Here's the drawing with two shaded views (mm, measured from the low corner). I have some questions. A direction names the side the tool comes from. Round coordinates to 2 decimals unless told otherwise and drop trailing zeros. Loops run counter-clockwise (first coordinate to the right, second up) from the corner with the lowest first, then second, coordinate; pieces in that order, holes last. Notation, with made-up numbers: (70, 2) -> (84, 2) arc R20 ccw to (84, 20) -> close; hole circle Ø2 at (84.5, 67.5). An arc over 180 degrees is marked (long way). Use a Markdown table: item, result.
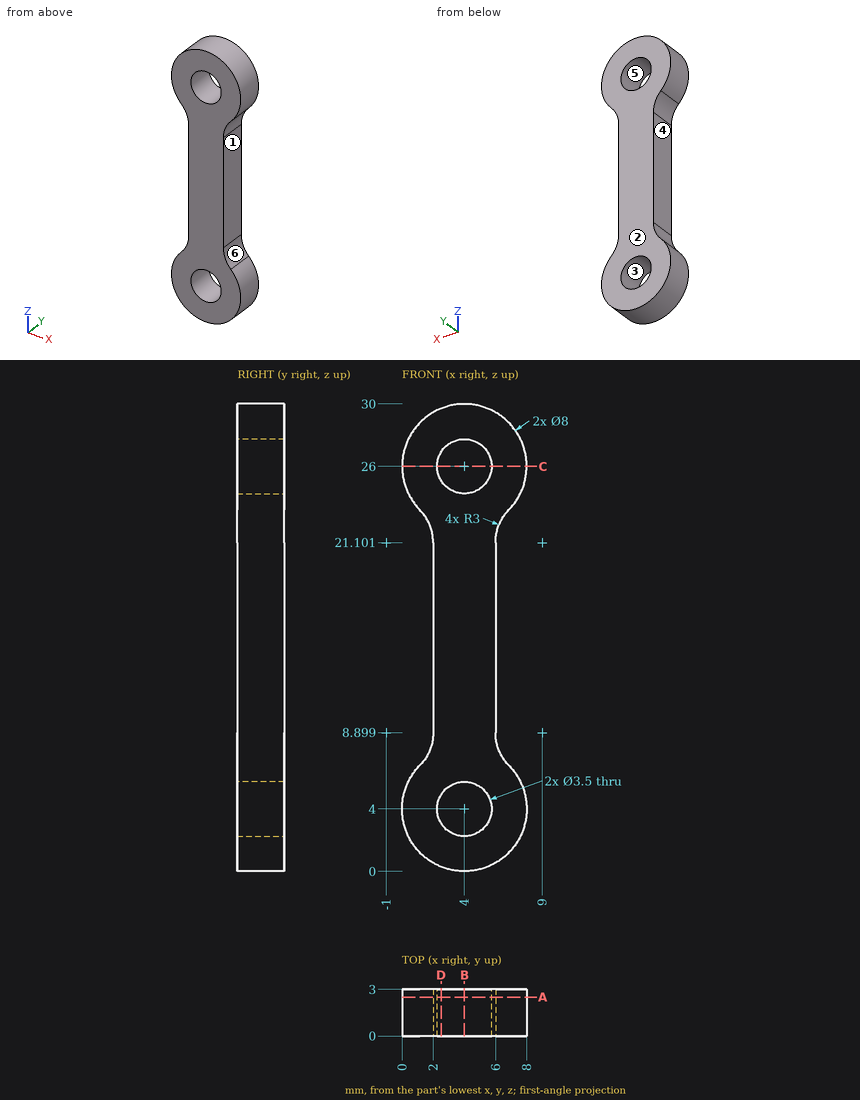
1. If we mould it in two halves opening along Z, with no side actions, what happens to the marked faces 1, 2 and 3? For each: +Z half, -Z half, draft (parallel to the pull), parting line (faces both ways), or undercut.
Answer sheet:
| item | result |
|---|---|
| face 1 | undercut |
| face 2 | draft |
| face 3 | undercut |
2. Which directions (+Z, -Z, +X, -X, +Y, -Y) give clear straight access to the entire face, cutting with the end or side of a thin tool? Please do the marked faces 4, 5 and 6.
Answer sheet:
| item | result |
|---|---|
| face 4 | -X, +Y, -Y |
| face 5 | +Y, -Y |
| face 6 | +X, +Y, -Y |
3. I want a section at C-C (z = 26). Please give me the cut outline in (x, y).
Answer sheet:
| item | result |
|---|---|
| outline | (0, 0) -> (2.25, 0) -> (2.25, 3) -> (0, 3) -> close; (5.75, 0) -> (8, 0) -> (8, 3) -> (5.75, 3) -> close |
4. I want a section at A-A (y = 2.5). Please give me the cut outline in (x, z).
Answer sheet:
| item | result |
|---|---|
| outline | (1.14, 6.8) arc R4 ccw (long way) to (6.86, 6.8) arc R3 cw to (6, 8.9) -> (6, 21.1) arc R3 cw to (6.86, 23.2) arc R4 ccw (long way) to (1.14, 23.2) arc R3 cw to (2, 21.1) -> (2, 8.9) arc R3 cw to start; hole circle Ø3.5 at (4, 4); hole circle Ø3.5 at (4, 26) |
5. I need wall thicknesses on line 1 (X direction, y = 1.8, z = 26); line 2 (Z direction, x = 5.25, y = 0.9); line 3 (X direction, y = 1.7, z = 17). Which ranges of each line are inside material? Lowest first, please.
Answer sheet:
| item | result |
|---|---|
| line 1 | x = 0 to 2.25, 5.75 to 8 |
| line 2 | z = 0.2 to 2.78, 5.22 to 24.78, 27.22 to 29.8 |
| line 3 | x = 2 to 6 |
6. I want a section at D-D (x = 2.5). Please give me the cut outline in (y, z).
Answer sheet:
| item | result |
|---|---|
| outline | (0, 0.29) -> (3, 0.29) -> (3, 3.1) -> (0, 3.1) -> close; (0, 4.9) -> (3, 4.9) -> (3, 25.1) -> (0, 25.1) -> close; (0, 26.9) -> (3, 26.9) -> (3, 29.71) -> (0, 29.71) -> close |
7. I want a section at B-B (x = 4). Please give me the cut outline in (y, z).
Answer sheet:
| item | result |
|---|---|
| outline | (0, 0) -> (3, 0) -> (3, 2.25) -> (0, 2.25) -> close; (0, 5.75) -> (3, 5.75) -> (3, 24.25) -> (0, 24.25) -> close; (0, 27.75) -> (3, 27.75) -> (3, 30) -> (0, 30) -> close |
8. Will these pins go through, and if not, where does the flat tip stop? pin 1 Ø0.9 at (y, z) = (2, 18) entering from +X; pin 2 Ø3 at (x, z) = (4, 26) entering from +Y.
Answer sheet:
| item | result |
|---|---|
| pin 1 | stops at x = 6 |
| pin 2 | passes through |
